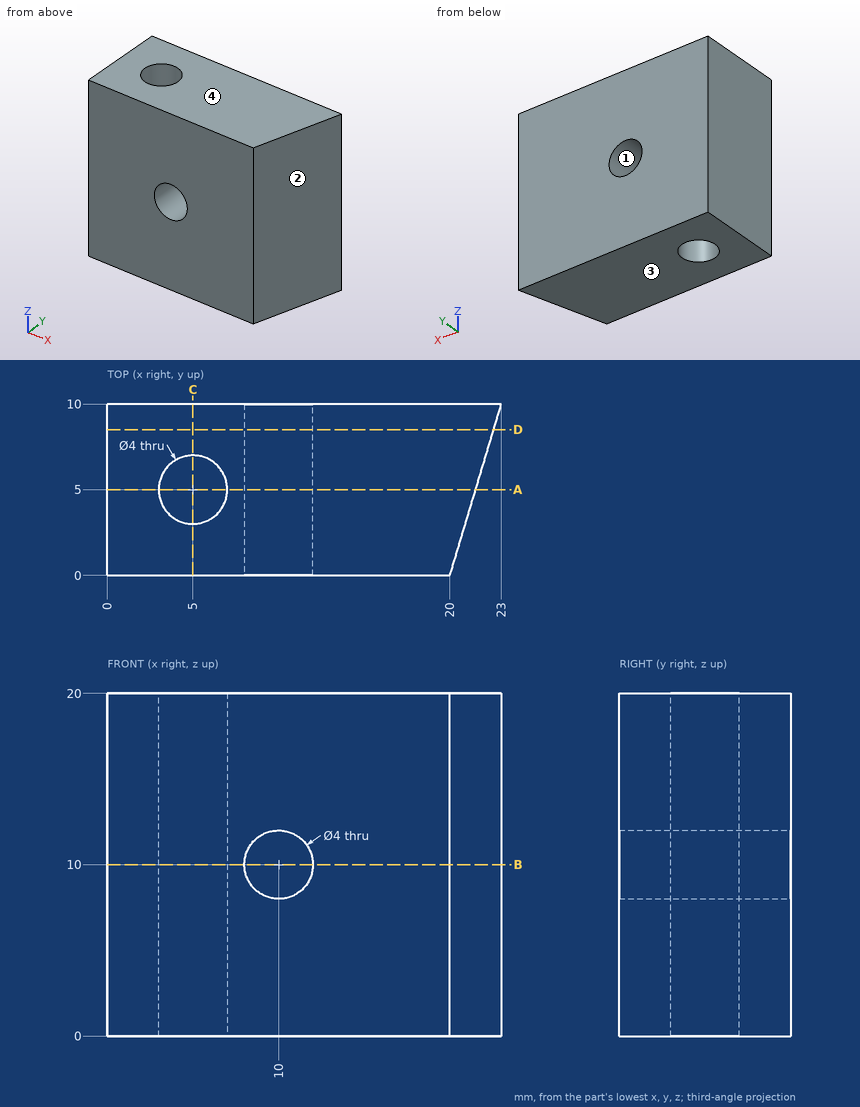
Drawing for the job (mm, zero at the part's lowest x, y, z). Coordinates: 2 decimals unless noted, no trailing zeros. Write each loop counter-clockwise with the first axis right and the second up, starting at its lowest first coordinate (ties: lowest second). Pieces come first, ordered by that corner, then holes. Notation, with made-up numbers: (59, -16.5) -> (71, -16.5) arc R17 ccw to (71, 7.5) -> close; hole circle Ø8 at (-33.5, 8). An arc over 180 degrees is marked (long way). One line per item, written item: value. Start each with the question number.
1) Slice it at C-C on x = 5. Write the cut outline in (y, z).
2) Slice it at A-A on y = 5. Write the cut outline in (x, z).
3) Pull direction Z, two halves, no side cores. Call the marked faces 1, 2, 3 and 4: +Z half, -Z half, draft (parallel to the pull), parting line (faces both ways), or undercut.
4) Probe probe 1 along Y at (x, z) = (5, 8.5); probe 2 along Z at (x, y) = (10, 4); probe 3 along X at (y, z) = (5.25, 9.25) (3 decimals). List the from-to ranges inside material, lowest first.
5) Slice it at D-D on y = 8.5. Write the cut outline in (x, z).
6) Flat gauge pin, fed straight in: pin 1 Ø3.5 at (x, y) = (5, 5) entering from +Z. Where does the tip first touch, or does it go through?
7) Slice it at B-B on z = 10. Write the cut outline in (x, y).
Answers follow:
1. outline: (0, 0) -> (3, 0) -> (3, 20) -> (0, 20) -> close; (7, 0) -> (10, 0) -> (10, 20) -> (7, 20) -> close
2. outline: (0, 0) -> (3, 0) -> (3, 20) -> (0, 20) -> close; (7, 0) -> (21.5, 0) -> (21.5, 20) -> (7, 20) -> close; hole circle Ø4 at (10, 10)
3. face 1: undercut
3. face 2: draft
3. face 3: -Z half
3. face 4: +Z half
4. probe 1: 0 to 3, 7 to 10
4. probe 2: 0 to 8, 12 to 20
4. probe 3: 0 to 3.016, 6.984 to 8.146, 11.854 to 21.575
5. outline: (0, 0) -> (22.55, 0) -> (22.55, 20) -> (0, 20) -> close; hole circle Ø4 at (10, 10)
6. pin 1: through
7. outline: (0, 0) -> (8, 0) -> (8, 10) -> (0, 10) -> close; (12, 0) -> (20, 0) -> (23, 10) -> (12, 10) -> close; hole circle Ø4 at (5, 5)
